from build123d import *

# Parameters (mm, degrees)
SKETCH1_W           = 115
SKETCH1_H           = 121
BOSS_EXTRUDE1_DEPTH = 10
BOSS_EXTRUDE2_DEPTH = 6
SKETCH3_R           = 12.5
SKETCH3_R_2         = 7
BOSS_EXTRUDE3_DEPTH = 3
SKETCH4_R           = 8.25
CUT_EXTRUDE1_DEPTH  = 6
SKETCH6_W           = 54.5
SKETCH6_H           = 50
BOSS_EXTRUDE5_DEPTH = 2
BOSS_EXTRUDE6_REACH = 117
CHAMFER1_SIZE       = 40


with BuildPart() as part:
    # Sketch1 → Boss-Extrude1 (new body)
    with BuildSketch(Plane(origin=(0, 0, 0), x_dir=(1, 0, 0), z_dir=(0, 1, 0))):
        Rectangle(SKETCH1_W, SKETCH1_H)
    extrude(amount=BOSS_EXTRUDE1_DEPTH)

    # Sketch2 → Boss-Extrude2 (add)
    with BuildSketch(Plane.XY.offset(60.5)):
        with BuildLine():
            Line((-12.5, 100), (-12.5, 0))
            Line((-12.5, 0), (12.5, 0))
            Line((12.5, 0), (12.5, 100))
            ThreePointArc((12.5, 100), (0, 112.5), (-12.5, 100))
        make_face()
    boss_extrude2 = extrude(amount=-BOSS_EXTRUDE2_DEPTH)

    # Sketch3 → Boss-Extrude3 (add)
    with BuildSketch(Plane(origin=(0, 0, 54.5), x_dir=(-1, 0, 0), z_dir=(0, 0, -1))):
        with Locations((0, 100)):
            Circle(SKETCH3_R)
        with Locations((0, 100)):
            Circle(SKETCH3_R_2, mode=Mode.SUBTRACT)
    boss_extrude3 = extrude(amount=BOSS_EXTRUDE3_DEPTH)

    # Sketch4 → Cut-Extrude1 (cut)
    with BuildSketch(Plane.XY.offset(60.5)):
        with Locations((0, 100)):
            Circle(SKETCH4_R)
    cut_extrude1 = extrude(amount=-CUT_EXTRUDE1_DEPTH, mode=Mode.SUBTRACT)

    # Sketch6 → Boss-Extrude5 (add, symmetric)
    with BuildSketch(Plane(origin=(0, 0, 0), x_dir=(0, 0, -1), z_dir=(1, 0, 0))):
        with Locations((-27.25, 35)):
            Rectangle(SKETCH6_W, SKETCH6_H)
    boss_extrude5 = extrude(amount=BOSS_EXTRUDE5_DEPTH, both=True)

    # Mirror1: Boss-Extrude2, Boss-Extrude3, Cut-Extrude1, Boss-Extrude5 across plane
    add(boss_extrude2.mirror(Plane.XY))
    add(boss_extrude3.mirror(Plane.XY))
    add(cut_extrude1.mirror(Plane.XY), mode=Mode.SUBTRACT)
    add(boss_extrude5.mirror(Plane.XY))

    # Sketch7 → Boss-Extrude6 (add, up to next)
    with BuildSketch(Plane.XY.offset(-54.5), mode=Mode.PRIVATE) as boss_extrude6_sk1:
        Polygon((2, 60), (12.5, 60), (2, 41.813466521), align=None)
    boss_extrude6_tool1 = extrude(boss_extrude6_sk1.sketch, amount=BOSS_EXTRUDE6_REACH, mode=Mode.PRIVATE) - part.part
    add(boss_extrude6_tool1.solids().sort_by_distance((5.5, 53.937822, -54.5))[0])
    # Sketch7 → Boss-Extrude6 (add, up to next)
    with BuildSketch(Plane.XY.offset(-54.5), mode=Mode.PRIVATE) as boss_extrude6_sk2:
        Polygon((-2, 60), (-12.5, 60), (-2, 41.813466521), align=None)
    boss_extrude6_tool2 = extrude(boss_extrude6_sk2.sketch, amount=BOSS_EXTRUDE6_REACH, mode=Mode.PRIVATE) - part.part
    add(boss_extrude6_tool2.solids().sort_by_distance((-5.5, 53.937822, -54.5))[0])

    # Chamfer1
    chamfer1_edges = [part.edges().sort_by_distance(p)[0] for p in [
        (57.5, 5, 60.5),
        (-57.5, 5, 60.5),
        (-57.5, 5, -60.5),
        (57.5, 5, -60.5),
    ]]
    chamfer(chamfer1_edges, length=CHAMFER1_SIZE)


solid = part.part
Could you check a few things on this model? Use its own coordinates, in mm. A direction names the side the tool comes from. Give positions to 0.01 mm unless a question says otherwise; leave off trailing zeros. Loops run counter-clockwise (first coordinate to the right, second up) from the corner with the lowest first, then second, coordinate; pieces in that order, holes last. Notation, with made-up numbers: (81, 55.25) -> (93, 55.25) arc R12 cw to (93, 71.25) -> close; hole circle Ø3 at (32.5, 80). An arc over 180 degrees is marked (long way). Answer as CSV lines item,"result". Start each with the question number.
(1) I need wall thicknesses on probe 1 along Y at (x, z) = (0, -52); probe 2 along Y at (x, z) = (0, -56.35); probe 3 along Z at (x, y) = (10, 24.5). Which ranges of each line are inside material? Lowest first, please.
(2) Which directions (+Z, -Z, +X, -X, +Y, -Y) give clear straight access to the entire face, cutting with the end or side of a thin tool? Please do faces 4 (the flat face through (-12.5, 56, 58)), 5 (the flat face through (23, 10, -1)), 6 (the flat face through (-7, 30, 54.5)), 7 (the flat face through (12.5, 54, 58)), 8 (the flat face through (-4, 94, -54.5)).
(3) If we section it at C-C on y = 35.5: Write out the boundary of the cut face in (x, z).
(4) If we section it at D-D on z = -6: Write out the boundary of the cut face in (x, y), then the cut area to 3 significant figures.
(5) If we section it at B-B on y = 68: Write out the boundary of the cut face in (x, z), then the cut area to 3 significant figures.
(6) I'm going to push flat-ended pins straight in: pin 1 Ø1.8 at (y, z) = (71.5, 56) entering from -X; pin 2 Ø3 at (y, z) = (45.5, 56.5) entering from +X; pin 3 Ø16.5 at (x, z) = (32.5, -7) entering from +Y. Where does each tip first touch, or does it pass through?
(7) We'd pull the mould along Y, two halves only. Please class faces 1 (the flat face through (7.32, 51.03, -0.76)), 2 (the cylindrical face through (0.91, 106.94, -53.02)), 3 (the flat face through (-37, 5, 41)): released by +Y, released by -Y, zero draft, split by the parting line, or undercut.
(8) If we section it at A-A on x = 0: Write out the boundary of the cut face in (y, z), then the cut area to 3 significant figures.
Computed:
1,probe 1,"y = 0 to 60, 87.5 to 93, 107 to 112.5"
1,probe 2,"y = 0 to 91.75, 108.25 to 112.5"
1,probe 3,"z = -60.5 to -54.5, 54.5 to 60.5"
2,face 4,"+Z, -Z, -X, +Y"
2,face 5,"+X"
2,face 6,"-X"
2,face 7,"+Z, -Z, +X, +Y"
2,face 8,"-Z"
3,outline,"(-12.5, -60.5) -> (12.5, -60.5) -> (12.5, -54.5) -> (2, -54.5) -> (2, 54.5) -> (12.5, 54.5) -> (12.5, 60.5) -> (-12.5, 60.5) -> (-12.5, 54.5) -> (-2, 54.5) -> (-2, -54.5) -> (-12.5, -54.5) -> close"
4,outline,"(-57.5, 0) -> (57.5, 0) -> (57.5, 10) -> (2, 10) -> (2, 41.81) -> (12.5, 60) -> (-12.5, 60) -> (-2, 41.81) -> (-2, 10) -> (-57.5, 10) -> close"
4,area,"1,540 mm2"
5,outline,"(-12.5, -60.5) -> (12.5, -60.5) -> (12.5, -54.5) -> (-12.5, -54.5) -> close; (-12.5, 54.5) -> (12.5, 54.5) -> (12.5, 60.5) -> (-12.5, 60.5) -> close"
5,area,"300 mm2"
6,pin 1,"stops at x = -12.5"
6,pin 2,"stops at x = 12.5"
6,pin 3,"stops at y = 10"
7,face 1,"undercut"
7,face 2,"undercut"
7,face 3,"zero draft"
8,outline,"(0, -60.5) -> (91.75, -60.5) -> (91.75, -54.5) -> (93, -54.5) -> (93, -51.5) -> (87.5, -51.5) -> (87.5, -54.5) -> (60, -54.5) -> (60, 54.5) -> (87.5, 54.5) -> (87.5, 51.5) -> (93, 51.5) -> (93, 54.5) -> (91.75, 54.5) -> (91.75, 60.5) -> (0, 60.5) -> close; (107, -54.5) -> (108.25, -54.5) -> (108.25, -60.5) -> (112.5, -60.5) -> (112.5, -51.5) -> (107, -51.5) -> close; (107, 51.5) -> (112.5, 51.5) -> (112.5, 60.5) -> (108.25, 60.5) -> (108.25, 54.5) -> (107, 54.5) -> close"
8,area,"7,760 mm2"
